Autodesk Inventor part; units mm, degrees
ref_plane "YZ Plane" through (0, 0, 0) normal (1, 0, 0) x (0, 1, 0)
ref_plane "XZ Plane" through (0, 0, 0) normal (0, 1, 0) x (-1, 0, 0)
ref_plane "XY Plane" through (0, 0, 0) normal (0, 0, 1) x (1, 0, 0)
sketch "スケッチ1" plane through (0, 0, 0) normal (0, 0, 1) x (1, 0, 0)
  line L0 (5, -5) -> (-5, -5)
  line L1 (-5, -5) -> (-5, 5)
  line L2 (-5, 5) -> (5, 5)
  line L3 (5, 5) -> (5, -5)
  line L4 (5, -5) -> (-5, 5) construction
  line L5 (-5, -5) -> (5, 5) construction
  line L6 (4, 4) -> (-4, 4)
  line L7 (-4, 4) -> (-4, -4)
  line L8 (-4, -4) -> (4, -4)
  line L9 (4, -4) -> (4, 4)
  point P0 (0, 0)
  dimension "d0" = 10
  dimension "d1" = 10
  dimension "d2" = 1
extrude "押し出し1" add sketch "スケッチ1" along normal blind 145
sketch "スケッチ2" plane through (5, -5, 0) normal (1, 0, 0) x (0, 0, -1)
  line L0 (0, 5) -> (-145, 5)
  line L1 (0, 1) -> (-145, 1)
  line L2 (0, 0) -> (0, 10)
  point P0 (-135, 5)
  point P1 (-10, 5)
  dimension "d5" = 10
  dimension "d6" = 125
hole "穴1" at (5, 0, 135) at (5, 0, 10) direction (-1, 0, 0) diameter 3.2 end through all
sketch "スケッチ3" plane through (-5, 5, 0) normal (0, 1, 0) x (1, 0, 0)
  line L0 (5, 0) -> (5, -145)
  line L1 (10, -145) -> (0, -145)
  line L2 (10, 0) -> (0, 0)
  point P0 (5, -125)
  point P1 (5, -20)
  point P2 (5, -89.5)
  point P3 (5, -72.5)
  dimension "d14" = 20
  dimension "d15" = 105
  dimension "d24" = 17
  dimension "d25" = 89.5
hole "穴2" at (0, 5, 125) at (0, 5, 20) at (0, 5, 89.5) direction (0, -1, 0) diameter 3.2 end through all
properties part number "kaku_1010_plate"
Model file for the job. Use its own axes, mm. A direction names the side the tool comes from. Give positions to 0.01 mm unless a question says otherwise; leave off trailing zeros. Order: outer loops, then holes, each group sorted by start corner. A loop starts at its lowest first (then second) coordinate and runs counter-clockwise, first axis right, second up. Notation, with made-up numbers: (53.5, 63.5) - (68.5, 63.5) arc R18 ccw to (68.5, 93.5) - close; hole circle Ø6 at (47.5, 4). An arc over 180 degrees is marked (long way). Write item = value, one per line. Start each with the question number.
1. Two-plate mould, pull along X, no slides. Class faces 1 (the flat face through (5, 0, 71)), 2 (the flat face through (0, -4, 71)), 3 (the cylindrical face through (-4.51, -0.07, 11.6)), 4 (the flat face through (4, 0, 71)): pulls with the +X half, pulls with the -X half, needs draft (parallel to the pull), parting line crosses it, or undercut.
2. Cut at D-D, the plane z = 135. List the corners of the cut face in (x, y), and give its area (3 significant figures).
3. Cut at B-B, the plane z = 118. List the corners of the cut face in (x, y), and give its area (3 significant figures).
4. Cut at A-A, the plane y = 0. List the corners of the cut face in (x, z).
5. Which spindle directions (+Z, -Z, +X, -X, +Y, -Y) get a long thin tool onto all of the face, cutting with end or side? Do faces 5 (the flat face through (-4, 0, 71)), 6 (the cylindrical face through (-1.08, -4.51, 18.82)). Say none if no direction does.
6. Probe line 1 along Z through (x, y) = (-4.65, 0); line 2 along Z through (x, y) = (0, 4.8); line 3 along X through (y, z) = (2.5, 47). List the from-to ranges inside material, lowest first.
7. Drop a flat-ended pin along its axis: P1, Ø2, axis at x = 0, z = 125, coming from the +Y side. Give the stop position or say it passes through.
8. Cut at C-C, the plane x = 0. State how many separate pieces and enclosed holes the cut face has, and give its area (3 significant figures).
Taken from the geometry:
q1.face_1 = pulls with the +X half
q1.face_2 = undercut
q1.face_3 = needs draft
q1.face_4 = undercut
q2.outline = (-5, -5) - (5, -5) - (5, -1.6) - (4, -1.6) - (4, -4) - (-4, -4) - (-4, -1.6) - (-5, -1.6) - close; (-5, 1.6) - (-4, 1.6) - (-4, 4) - (4, 4) - (4, 1.6) - (5, 1.6) - (5, 5) - (-5, 5) - close
q2.area = 29.6 mm²
q3.outline = (-5, -5) - (5, -5) - (5, 5) - (-5, 5) - close; hole (-4, -4) - (4, -4) - (4, 4) - (-4, 4) - close
q3.area = 36.0 mm²
q4.outline = (-5, 0) - (-4, 0) - (-4, 8.4) - (-5, 8.4) - close; (-5, 11.6) - (-4, 11.6) - (-4, 133.4) - (-5, 133.4) - close; (-5, 136.6) - (-4, 136.6) - (-4, 145) - (-5, 145) - close; (4, 0) - (5, 0) - (5, 8.4) - (4, 8.4) - close; (4, 11.6) - (5, 11.6) - (5, 133.4) - (4, 133.4) - close; (4, 136.6) - (5, 136.6) - (5, 145) - (4, 145) - close
q5.face_5 = +Z, -Z
q5.face_6 = +Y, -Y
q6.line_1 = 0 to 8.4, 11.6 to 133.4, 136.6 to 145
q6.line_2 = 0 to 18.4, 21.6 to 87.9, 91.1 to 123.4, 126.6 to 145
q6.line_3 = -5 to -4, 4 to 5
q7.P1 = through
q8.separate_pieces = 8
q8.enclosed_holes = 0
q8.area = 271 mm²
